from build123d import *

# Parameters (mm, degrees)
F1_DEPTH = 12
F2_SIZE2 = 10
F2_SIZE  = 1.2


with BuildPart() as f1:
    # F0 (on Top) → F1 (new body)
    with BuildSketch(Plane.XY):
        with BuildLine():
            Line((35, 21), (-35, 21))
            ThreePointArc((-35, 21), (-56, 0), (-35, -21))
            Line((-35, -21), (35, -21))
            ThreePointArc((35, -21), (56, 0), (35, 21))
        make_face()
        with BuildLine():
            Line((35, -19), (-35, -19))
            ThreePointArc((-35, -19), (-54, 0), (-35, 19))
            Line((-35, 19), (35, 19))
            ThreePointArc((35, 19), (54, 0), (35, -19))
        make_face(mode=Mode.SUBTRACT)
    extrude(amount=F1_DEPTH)

    # F2
    f2_edges = [f1.edges().sort_by_distance(p)[0] for p in [
        (0, -19, 0),
    ]]
    f2_side = f1.faces().sort_by_distance((0, 19.803839, 0))[0]
    chamfer(f2_edges, length=F2_SIZE, length2=F2_SIZE2, reference=f2_side)


solid = f1.part
Here's how the part is built. I have some questions about the finished solid (model axes, mm). A direction names the side the tool comes from. Coordinates: 2 decimals unless noted, no trailing zeros. Write each loop counter-clockwise with the first axis right and the second up, starting at its lowest first coordinate (ties: lowest second). Pieces come first, ordered by that corner, then holes.
Item 1: On a 3-axis mill with a long thin cutter (end or side, diameter ignored), from which of +Z, -Z, +X, -X, +Y, -Y can I reach the whole of each face in a straight line? I mean faces 5 (the flat face through (-0.49, 19.59, 5.07)), 6 (the flat face through (0, -19, 11)), 7 (the flat face through (0, 21, 6)). Say none if no direction works.
Item 2: If we mould it in two halves opening along X, with no side actions, what happens to faces 1 (the cylindrical face through (-54, 0, 11)), 2 (the cylindrical face through (56, 0, 6)), 3 (the cylindrical face through (-56, 0, 6)), 4 (the cylindrical face through (54, 0, 11))? For each: +X half, -X half, draft (parallel to the pull), parting line (faces both ways), or undercut.
Item 3: I want a section at B-B on x = -9. Write out the boundary of the cut face in (y, z), and give its area (3 significant figures).
Item 4: I want a section at D-D on z = 1. Write out the boundary of the cut face in (x, y), and give its area (3 significant figures).
Item 5: I want a section at C-C on z = 7. Write out the boundary of the cut face in (x, y).
Item 6: If I drill on line 1 (Y direction, x = 30.5, z = 2.5); line 2 (Y direction, x = -35, z = 5.25); line 3 (X direction, y = 16.5, z = 2.5), over which ranges is the centre line in solid material (lowest first)?
Item 7: I want a section at A-A on y = 0. Write out the boundary of the cut face in (x, z), and give its area (3 significant figures).
Item 8: Will these pins go through, and if not, where does the flat tip stop? pin 1 (3 mm diameter, centred on y = -10, z = 9.5, fed in from -X); pin 2 (4 mm diameter, centred on y = -14, z = 1.5, fed in from -X).
Findings below:
1. face 5: -Z
1. face 6: +Z, -Z
1. face 7: +Z, -Z, +X, -X, +Y
2. face 1: undercut
2. face 2: +X half
2. face 3: -X half
2. face 4: undercut
3. outline: (-21, 0) - (-20.2, 0) - (-19, 10) - (-19, 12) - (-21, 12) - close; (19, 10) - (20.2, 0) - (21, 0) - (21, 12) - (19, 12) - close
3. area: 36.0 mm2
4. outline: (-35, -21) - (35, -21) arc R21 ccw to (35, 21) - (-35, 21) arc R21 ccw to start; hole (-35, -20.08) - (35, -20.08) arc R20.08 ccw to (35, 20.08) - (-35, 20.08) arc R20.08 ccw to start
4. area: 248 mm2
5. outline: (-35, -21) - (35, -21) arc R21 ccw to (35, 21) - (-35, 21) arc R21 ccw to start; hole (-35, -19.36) - (35, -19.36) arc R19.36 ccw to (35, 19.36) - (-35, 19.36) arc R19.36 ccw to start
6. line 1: y = -21 to -19.9, 19.9 to 21
6. line 2: y = -21 to -19.57, 19.57 to 21
6. line 3: x = -47.99 to -46.12, 46.12 to 47.99
7. outline: (-56, 0) - (-55.2, 0) - (-54, 10) - (-54, 12) - (-56, 12) - close; (54, 10) - (55.2, 0) - (56, 0) - (56, 12) - (54, 12) - close
7. area: 36.0 mm2
8. pin 1: stops at x = -54.2
8. pin 2: stops at x = -52.23
